Autodesk Inventor part; units mm, degrees
ref_plane "YZ Plane" through (0, 0, 0) normal (1, 0, 0) x (0, 1, 0)
ref_plane "XZ Plane" through (0, 0, 0) normal (0, 1, 0) x (-1, 0, 0)
ref_plane "XY Plane" through (0, 0, 0) normal (0, 0, 1) x (1, 0, 0)
sketch "Sketch1" plane through (0, 0, 0) normal (0, 1, 0) x (-1, 0, 0)
  circle A0 centre (80, -20) radius 1.5
  circle A1 centre (80, -40) radius 1.5
  circle A2 centre (80, -60) radius 1.5
  circle A3 centre (80, -80) radius 1.5
  circle A4 centre (60, -80) radius 1.5
  circle A5 centre (60, -60) radius 1.5
  circle A6 centre (60, -40) radius 1.5
  circle A7 centre (60, -20) radius 1.5
  circle A8 centre (20, -60) radius 1.5
  circle A9 centre (20, -40) radius 1.5
  circle A10 centre (40, -60) radius 1.5
  circle A11 centre (40, -40) radius 1.5
  circle A12 centre (50, -50) radius 1.5
  line L0 (82.9894, -14.3145) -> (14.4573, -14.3145)
  line L1 (14.4573, -14.3145) -> (14.4573, -84.9883)
  line L2 (14.4573, -84.9883) -> (82.9894, -84.9883)
  line L3 (82.9894, -84.9883) -> (82.9894, -14.3145)
  point P0 (0, 0)
  dimension "d4" = 3
  dimension "d5" = 3
  dimension "d6" = 3
  dimension "d7" = 3
  dimension "d8" = 3
  dimension "d9" = 3
  dimension "d10" = 3
  dimension "d11" = 3
  dimension "d13" = 3
  dimension "d14" = 3
  dimension "d15" = 3
  dimension "d16" = 3
  dimension "d17" = 60
  dimension "d20" = 3
extrude "Extrusion1" add sketch "Sketch1" along normal blind 3
chamfer "Chamfer1" distance 2 angle 45 4 edges at (-14.4573, 1.5, -14.3145) (-14.4573, 1.5, -84.9883) (-82.9894, 1.5, -84.9883) (-82.9894, 1.5, -14.3145)
sketch "Sketch2" plane through (0, 0, 0) normal (0, -1, 0) x (1, 0, 0)
  line L0 (-14.4573, -16.3145) -> (-14.4573, -82.9883)
  line L1 (-14.4573, -82.9883) -> (-14.4573, -74.9883)
  line L2 (-16.4573, -84.9883) -> (-80.9894, -84.9883)
  line L3 (-16.4573, -84.9883) -> (-24.4573, -84.9883)
  line L4 (-24.4573, -84.9883) -> (-14.4573, -74.9883)
  line L5 (-16.4573, -84.9883) -> (-14.4573, -82.9883)
  line L6 (-16.4573, -84.9883) -> (-14.4573, -82.9883)
  line L7 (-80.9894, -84.9883) -> (-72.9894, -84.9883)
  line L8 (-82.9894, -82.9883) -> (-82.9894, -16.3145)
  line L9 (-80.9894, -84.9883) -> (-82.9894, -82.9883)
  line L10 (-82.9894, -82.9883) -> (-82.9894, -74.9883)
  line L11 (-82.9894, -74.9883) -> (-72.9894, -84.9883)
  line L12 (-80.9894, -14.3145) -> (-16.4573, -14.3145)
  line L13 (-16.4573, -14.3145) -> (-24.4573, -14.3145)
  line L14 (-16.4573, -14.3145) -> (-14.4573, -16.3145)
  line L15 (-14.4573, -16.3145) -> (-14.4573, -24.3145)
  line L16 (-14.4573, -24.3145) -> (-24.4573, -14.3145)
  line L17 (-82.9894, -16.3145) -> (-82.9894, -24.3145)
  line L18 (-82.9894, -16.3145) -> (-80.9894, -14.3145)
  line L19 (-80.9894, -14.3145) -> (-72.9894, -14.3145)
  line L20 (-72.9894, -14.3145) -> (-82.9894, -24.3145)
  point P0 (0, 0)
  dimension "d26" = 8
  dimension "d27" = 8
  dimension "d28" = 8
  dimension "d29" = 8
  dimension "d30" = 8
  dimension "d31" = 8
  dimension "d32" = 8
  dimension "d33" = 8
extrude "Extrusion2" add sketch "Sketch2" along normal blind 8 contours L0 L16 L12 L14 | L0 L5 L2 L4 | L20 L8 L18 L12 | L2 L9 L8 L11
extrude "Extrusion3" cut sketch "Sketch1" against normal blind 3 contours A0 | A3
fillet "Fillet1" radius 1 1 edges at (-82.9894, -4, -24.3145)
fillet "Fillet2" radius 1 7 edges at (-72.9894, -4, -14.3145) (-14.4573, -4, -24.3145) (-14.4573, -4, -74.9883) (-24.4573, -4, -84.9883) (-72.9894, -4, -84.9883) (-24.4573, -4, -14.3145) (-82.9894, -4, -74.9883)
chamfer "Chamfer2" distance 0.2 angle 45 13 edges at (-78.5, 3, -80) (-58.5, 3, -80) (-58.5, 3, -60) (-78.5, 3, -60) (-38.5, 3, -60) (-18.5, 3, -60) (-18.5, 3, -40) (-38.5, 3, -40) (-48.5, 3, -50) (-58.5, 3, -40) (-58.5, 3, -20) (-78.5, 3, -40) (-78.5, 3, -20)
chamfer "Chamfer3" distance 1 angle 45 8 edges at (-48.7233, 3, -14.3145) (-14.4573, 3, -49.6514) (-48.7233, 3, -84.9883) (-82.9894, 3, -49.6514) (-81.9894, 3, -83.9883) (-15.4573, 3, -83.9883) (-15.4573, 3, -15.3145) (-81.9894, 3, -15.3145)
sketch "Sketch4" plane through (0, 3, 0) normal (0, 1, 0) x (1, 0, 0)
  point P0 (0, 0)
equation "\"BendRadius\" = Thickness"
equation "\"BendReliefWidth\" = Thickness"
equation "\"BendReliefDepth\" = 0.5 * Thickness"
equation "\"CornerReliefSize\" = 4 * Thickness"
equation "\"MinimumRemnant\" = 2 * Thickness"
equation "\"TransitionRadius\" = BendRadius"
equation "\"JacobiRadiusSize\" = BendRadius"
equation "\"GapSize\" = Thickness"
properties part number "Repick"
Geometry: final body of the model. Coordinates: model frame, mm. A direction names the side the tool comes from. Round coordinates to 2 decimals unless told otherwise and drop trailing zeros. Order: outer loops, then holes, each group sorted by start corner. A loop starts at its lowest first (then second) coordinate and runs counter-clockwise, first axis right, second up. Notation, with made-up numbers: M 59,37 L 70,37 A12 ccw 70,48 Z; hole C 12,81 d3. An arc over 180 degrees is marked long. Use one line per item in the form item = value. Start each with the question number.
Q1. Pin query (flat end, axial travel): pin 1 Ø4 at (x, z) = (-50, -50) entering from -Y; pin 2 Ø0.9 at (x, z) = (-80, -80) entering from +Y; pin 3 Ø1.8 at (x, z) = (-60, -80) entering from -Y. Return the tip coordinate at first contact, or that it passes through.
Q2. Material intervals for line 1 (Z direction, x = -20, y = 1.2); line 2 (Y direction, x = -78, z = -31); line 3 (Z direction, x = -51, y = 2), sorted ascending. Write a range as [from, to].
Q3. Mould query, pull axis Z, two halves, no side actions, for faces 1 (the face through (-81.655, 2.493, -83.626)), 2 (the face through (-15.792, 2.493, -15.677)), 3 (the face through (-80.69, 1.38, -38.67)). Classes: +Z half, -Z half, draft (parallel to the pull), parting line (faces both ways), or undercut.
Q4. Cut plane B-B (y = -4.5). Return loops of the section in (x, z), and give its area (3 significant figures).
Q5. Cut plane C-C (x = -50). Return loops of the section in (y, z).
Q6. Access query for faces 4 (the face through (-80, -3, -20)), 5 (the face through (-82.989, 0.3, -50.1)), 6 (the face through (-74.49, -4.06, -84.39)). Directions: +Z, -Z, +X, -X, +Y, -Y. A direction counts if a zero-diameter tool reaches every point of the face in a straight line with its end or side. Return the directions, or none.
Q7. Cut plane A-A (x = -40). Return loops of the section in (y, z).
Q8. Cut plane D-D (z = -75). Return loops of the section in (x, y), and give its area (3 significant figures).
Geometry results:
q1.pin_1 = 0
q1.pin_2 = -3
q1.pin_3 = through
q2.line_1 = [-84.99, -61.5], [-58.5, -41.5], [-38.5, -14.31]
q2.line_2 = [0, 3]
q2.line_3 = [-84.99, -51.12], [-48.88, -14.31]
q3.face_1 = -Z half
q3.face_2 = +Z half
q3.face_3 = undercut
q4.outline = M -82.99,-82.99 L -80.99,-84.99 L -75.4,-84.99 A1 ccw -74.7,-83.28 L -81.28,-76.7 A1 ccw -82.99,-77.4 Z; M -82.99,-21.9 A1 ccw -81.28,-22.61 L -74.7,-16.02 A1 ccw -75.4,-14.31 L -80.99,-14.31 L -82.99,-16.31 Z; M -22.75,-83.28 A1 ccw -22.04,-84.99 L -16.46,-84.99 L -14.46,-82.99 L -14.46,-77.4 A1 ccw -16.16,-76.7 Z; M -22.75,-16.02 L -16.16,-22.61 A1 ccw -14.46,-21.9 L -14.46,-16.31 L -16.46,-14.31 L -22.04,-14.31 A1 ccw Z
q4.area = 182 mm^2
q5.outline = M 0,-84.99 L 2,-84.99 L 3,-83.99 L 3,-51.7 L 2.8,-51.5 L 0,-51.5 Z; M 0,-48.5 L 2.8,-48.5 L 3,-48.3 L 3,-15.31 L 2,-14.31 L 0,-14.31 Z
q6.face_4 = +Y
q6.face_5 = +Z, -Z, -X, +Y, -Y
q6.face_6 = -Y
q7.outline = M 0,-84.99 L 2,-84.99 L 3,-83.99 L 3,-61.7 L 2.8,-61.5 L 0,-61.5 Z; M 0,-58.5 L 2.8,-58.5 L 3,-58.3 L 3,-41.7 L 2.8,-41.5 L 0,-41.5 Z; M 0,-38.5 L 2.8,-38.5 L 3,-38.3 L 3,-15.31 L 2,-14.31 L 0,-14.31 Z
q8.outline = M -82.99,0 L -14.46,0 L -14.46,2 L -15.46,3 L -81.99,3 L -82.99,2 Z
q8.area = 205 mm^2
